Here's how the part is built. I have some questions about the finished solid (model axes, mm). A direction names the side the tool comes from. Coordinates: 2 decimals unless noted, no trailing zeros. Loops run counter-clockwise (first coordinate to the right, second up) from the corner with the lowest first, then second, coordinate; pieces in that order, holes last. Notation, with made-up numbers: (41.25, -25) -> (86.25, -25) arc R22 ccw to (86.25, -7) -> close; hole circle Ø3 at (15.5, 85.25). An arc over 180 degrees is marked (long way). Use CSV: the item, a comma, the result in double quotes. Start each with the question number.
from build123d import *

# Parameters (mm, degrees)
SKETCH1_W               = 8
SKETCH1_H               = 8
BOSS_EXTRUDE1_DEPTH     = 3
CUT_EXTRUDE1_DEPTH      = 12.704699911
CUT_EXTRUDE1_DEPTH_BACK = 12.704699911
CUT_EXTRUDE2_DEPTH      = 11
SKETCH4_R               = 1.8
CUT_EXTRUDE3_DEPTH      = 0.8
SKETCH5_W               = 8
SKETCH5_H               = 1
BOSS_EXTRUDE2_DEPTH     = 2
FILLET1_R               = 4
CUT_EXTRUDE4_DEPTH      = 0.4


with BuildPart() as part:
    # Sketch1 → Boss-Extrude1 (new body)
    with BuildSketch(Plane(origin=(0, 0, 0), x_dir=(1, 0, 0), z_dir=(0, 1, 0))):
        with Locations((4, 4)):
            Rectangle(SKETCH1_W, SKETCH1_H)
    extrude(amount=BOSS_EXTRUDE1_DEPTH)

    # Sketch2 → Cut-Extrude1 (cut, two sides: drawn at the far end of the back side and taken through both)
    with BuildSketch(Plane.XY.offset(-CUT_EXTRUDE1_DEPTH_BACK)):
        Polygon((0, 0), (0.6, 3), (0, 3), align=None)
        Polygon((8, 0), (7.4, 3), (8, 3), align=None)
    extrude(amount=CUT_EXTRUDE1_DEPTH + CUT_EXTRUDE1_DEPTH_BACK, mode=Mode.SUBTRACT)

    # Sketch3 → Cut-Extrude2 (cut)
    with BuildSketch(Plane(origin=(0, 0, 0), x_dir=(0, 0, -1), z_dir=(1, 0, 0))):
        Polygon((0, 0), (0.6, 3), (0, 3), align=None)
        Polygon((8, 3), (7.4, 3), (8, 0), align=None)
    extrude(amount=CUT_EXTRUDE2_DEPTH, mode=Mode.SUBTRACT)

    # Sketch4 → Cut-Extrude3 (cut)
    with BuildSketch(Plane.XZ):
        with Locations(Location((4, -3.75, 0), (0, 0, 270))):
            Circle(SKETCH4_R)
    extrude(amount=-CUT_EXTRUDE3_DEPTH, mode=Mode.SUBTRACT)

    # Sketch5 → Boss-Extrude2 (add)
    with BuildSketch(Plane.XZ):
        with Locations((4, -7.5)):
            Rectangle(SKETCH5_W, SKETCH5_H)
    extrude(amount=BOSS_EXTRUDE2_DEPTH)

    # Fillet1
    # the kernel refuses this fillet: 4 mm, written as the material it takes off along each edge
    with BuildSketch(Plane(origin=(8, -2, -16.660254038), x_dir=(0, 1, 0), z_dir=(0, 0, 1)), Plane(origin=(0, -2, 1.660254038), x_dir=(0, 1, 0), z_dir=(0, 0, -1))) as fillet1_piece_1:
        with BuildLine():
            CenterArc((4, 3.464101615), FILLET1_R, 180, 60)
            Line((0, 3.464101615), (-0.08, 3.464101615))
            Line((-0.08, 3.464101615), (-0.08, 0))
            Line((-0.08, 0), (0, -0.08))
            ThreePointArc((0, -0.08), (1, -0.08), (1.96, -0.069282032))
            Line((1.96, -0.069282032), (2, 0))
        make_face()
    extrude(amount=18.320508076, mode=Mode.SUBTRACT)

    # Sketch6 → Cut-Extrude4 (cut)
    with BuildSketch(Plane(origin=(0, 3, 0), x_dir=(1, 0, 0), z_dir=(0, 1, 0))):
        Polygon((2.030290665, 2.010567225), (2.030290665, 6.010567225), (3.331572716, 6.010567225), (4.004649639, 3.28220184), (4.677726562, 6.010567225), (5.979008613, 6.010567225), (5.979008613, 2.010567225), (5.209777844, 2.010567225), (5.184136818, 5.159605686), (4.433335536, 2.010567225), (3.575963742, 2.010567225), (2.82516246, 5.159605686), (2.799521434, 2.010567225), align=None)
    extrude(amount=-CUT_EXTRUDE4_DEPTH, mode=Mode.SUBTRACT)


solid = part.part
1) Please list where these lines run through material, in increasing order: L1, parallel to Y at x = 2.5, z = -5.25; L2, parallel to X at y = 0.6, z = -3.75; L3, parallel to Y at x = 5, z = -4. Write a range as [from, to].
2) I want a section at D-D, the plane y = 1.3. Please give me the cut outline in (x, z).
3) I want a section at B-B, the plane x = 4.25. Please give me the cut outline in (y, z), plus the area to 3 significant figures.
4) I want a section at C-C, the plane z = -3.75. Please give me the cut outline in (x, y).
5) Which directions (+Z, -Z, +X, -X, +Y, -Y) give clear straight access to the entire face, cutting with the end or side of a thin tool? Please do faces 1 (the face through (3, 0, -2)), 2 (the face through (1.49, -1.48, -7.49)), 3 (the face through (4, 0.8, -4)), 4 (the face through (4.5, 2.6, -4)).
6) For P1, Ø2, axis at x = 5, y = 2.5, coming from the +Z side; P2, Ø3, axis at x = 4, z = -3.5, coming from the -Y side, each with a flat end and sliding along its axis, tell me the tip position at first contact or that it passes through.
7) I want a section at A-A, the plane y = 0.35. Please give me the cut outline in (x, z), plus the area to 3 significant figures.
8) Thinking about a two-plate mould opening in X: for faces 5 (the face through (0.3, 1.5, -4.1)), 6 (the face through (4.541, 0.394, -5.467)), 7 (the face through (4, -2, -7.5)), which applies, pulls with the +X half, pulls with the -X half, needs draft (parallel to the pull), parting line crosses it, or undercut?
Return value:
1,L1,"y = [0, 2.6]"
1,L2,"x = [0.12, 2.2], [5.8, 7.88]"
1,L3,"y = [0.8, 3]"
2,outline,"(0.26, -7.74) -> (7.74, -7.74) -> (7.74, -0.26) -> (0.26, -0.26) -> close"
3,outline,"(-2, -8) -> (0, -8) -> (3, -7.4) -> (3, -4.28) -> (2.6, -4.28) -> (2.6, -2.01) -> (3, -2.01) -> (3, -0.6) -> (0, 0) -> (0, -1.97) -> (0.8, -1.97) -> (0.8, -5.53) -> (0, -5.53) -> (0, -7) -> (-2, -7) -> close"
3,area,"20.4 mm²"
4,outline,"(0, 0) -> (2.2, 0) -> (2.2, 0.8) -> (5.8, 0.8) -> (5.8, 0) -> (8, 0) -> (7.4, 3) -> (5.98, 3) -> (5.98, 2.6) -> (5.2, 2.6) -> (5.2, 3) -> (4.85, 3) -> (4.85, 2.6) -> (4.12, 2.6) -> (4.12, 3) -> (3.89, 3) -> (3.89, 2.6) -> (3.16, 2.6) -> (3.16, 3) -> (2.81, 3) -> (2.81, 2.6) -> (2.03, 2.6) -> (2.03, 3) -> (0.6, 3) -> close"
5,face 1,"+Z, +X, -X, -Y"
5,face 2,"+Z, -Z, -X, -Y"
5,face 3,"-Y"
5,face 4,"+Y"
6,P1,"stops at z = -0.3"
6,P2,"stops at y = 0.8"
7,outline,"(0.07, -7.93) -> (7.93, -7.93) -> (7.93, -0.07) -> (0.07, -0.07) -> close; hole circle Ø3.6 at (4, -3.75)"
7,area,"51.6 mm²"
8,face 5,"pulls with the -X half"
8,face 6,"undercut"
8,face 7,"needs draft"
